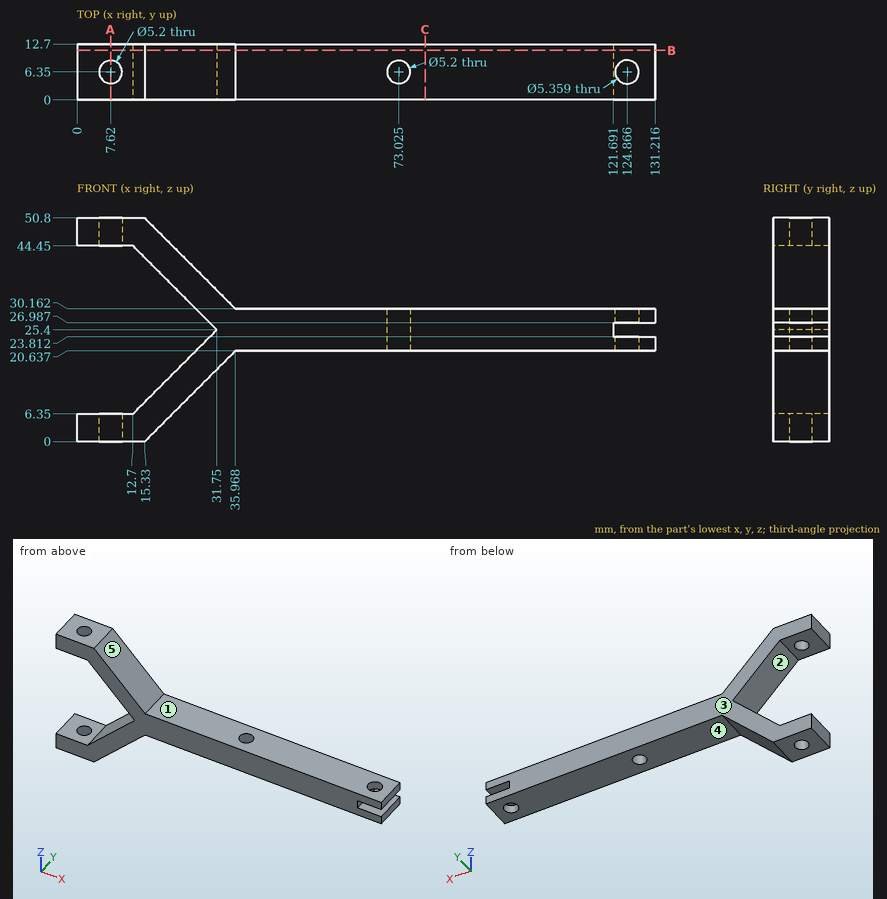
Could you check a few things on this drawing? It's one solid part, dimensions in mm from its lowest x, y, z. A direction names the side the tool comes from. Coordinates: 2 decimals unless noted, no trailing zeros. Write each loop counter-clockwise with the first axis right and the second up, starting at its lowest first coordinate (ties: lowest second). Pieces come first, ordered by that corner, then holes. Notation, with made-up numbers: (-2.5, 33.5) - (34.5, 33.5) arc R31 cw to (34.5, 66.5) - close; hole circle Ø2 at (-21, 41.5). An arc over 180 degrees is marked (long way). Use one line per item in the form item = value.
1) I need wall thicknesses on line 1 (Y direction, x = 7.62, z = 4.5); line 2 (Z direction, x = 101, y = 9.5); line 3 (Z direction, x = 19.5, y = 2). Which ranges of each line are inside material? Lowest first, please.
Solved:
line_1 = 0 to 3.75, 8.95 to 12.7
line_2 = 20.64 to 30.16
line_3 = 4.17 to 13.15, 37.65 to 46.63
2) Suppose I cut it at C-C, the plane x = 79. Write out the boundary of the cut face in (y, z), plus the area to 3 significant figures.
Solved:
outline = (0, 20.64) - (12.7, 20.64) - (12.7, 30.16) - (0, 30.16) - close
area = 121 mm2
3) I'm going to push flat-ended pins straight in: P1, Ø3, axis at x = 127, y = 6.5, coming from the +Z side; P2, Ø4, axis at x = 7.62, y = 6.35, coming from the -Z side; P3, Ø2.5, axis at y = 4, z = 25.5, coming from the +X side; P4, Ø6, axis at x = 73.025, y = 6.35, coming from the -Z side. Where does each tip first touch, or does it pass through?
Solved:
P1 = 30.16
P2 = through
P3 = 121.69
P4 = 20.64
4) Thinking about a two-plate mould opening in Z: for the marked faces 1, 2 and 3, which applies, released by +Z, released by -Z, zero draft, split by the parting line, or undercut?
Solved:
face_1 = released by +Z
face_2 = undercut
face_3 = zero draft
5) Suppose I cut it at B-B, the plane y = 11.25. Write out the boundary of the cut face in (x, z), plus the area to 3 significant figures.
Solved:
outline = (0, 0) - (15.33, 0) - (35.97, 20.64) - (131.22, 20.64) - (131.22, 23.81) - (121.69, 23.81) - (121.69, 26.99) - (131.22, 26.99) - (131.22, 30.16) - (35.97, 30.16) - (15.33, 50.8) - (0, 50.8) - (0, 44.45) - (12.7, 44.45) - (31.75, 25.4) - (12.7, 6.35) - (0, 6.35) - close
area = 1,430 mm2
6) On a 3-axis mill with a long thin cutter (end or side, diameter ignored), from which of +Z, -Z, +X, -X, +Y, -Y can I reach the whole of each face in a straight line? I mean the marked faces 4 and 5. Say none if no direction works.
Solved:
face_4 = -Z, +X, +Y, -Y
face_5 = +Z, +X, +Y, -Y
7) Suppose I cut it at A-A, the plane x = 7.62. Write out the boundary of the cut face in (y, z).
Solved:
outline = (0, 0) - (3.75, 0) - (3.75, 6.35) - (0, 6.35) - close; (0, 44.45) - (3.75, 44.45) - (3.75, 50.8) - (0, 50.8) - close; (8.95, 0) - (12.7, 0) - (12.7, 6.35) - (8.95, 6.35) - close; (8.95, 44.45) - (12.7, 44.45) - (12.7, 50.8) - (8.95, 50.8) - close
